Input: dimensioned drawing with shaded views. Units: mm. Origin: part minimum x, y, z. A direction names the side the tool comes from. Coordinates: 2 decimals unless noted, no trailing zeros. Order: outer loops, then holes, each group sorted by start corner. A loop starts at its lowest first (then second) coordinate and runs counter-clockwise, first axis right, second up. Notation, with made-up numbers: (2, 41.25) -> (51, 41.25) arc R31 cw to (51, 75.25) -> close; hole circle Ø3 at (-11.75, -4.75). An arc over 180 degrees is marked (long way). Write item = value, one per line. Start each with the question number.
Item 1: Set-up query: the marked faces 1 and 2. Return all of +Z, -Z, +X, -X, +Y, -Y with unobstructed straight access to the full face (end or side cutting, diameter ignored); none if empty.
Item 2: Section query B-B (x = 36). Output: boundary loops of the cut face in (y, z), then the cut area to 3 significant figures.
Item 3: Ray query, line 1 along Z through (x, y) = (36, 2); line 2 along Y through (x, z) = (2.35, 10). Return the intervals inside material, ascending. Write a range as [from, to].
Item 4: Section query D-D (z = 45). Output: boundary loops of the cut face in (x, y), then the cut area to 3 significant figures.
Item 5: Contact query for flat-ended pins moving along their axis: pin 1 (4 mm diameter, centred on x = 36, z = 40, fed in from +Y) (3 decimals); pin 2 (8.5 mm diameter, centred on y = 36, z = 10, fed in from +X); pin 3 (1 mm diameter, centred on x = 26, z = 39.5, fed in from +Y). Output: stop coordinate, or through.
Item 6: Section query A-A (z = 10). Output: boundary loops of the cut face in (x, y), then the cut area to 3 significant figures.
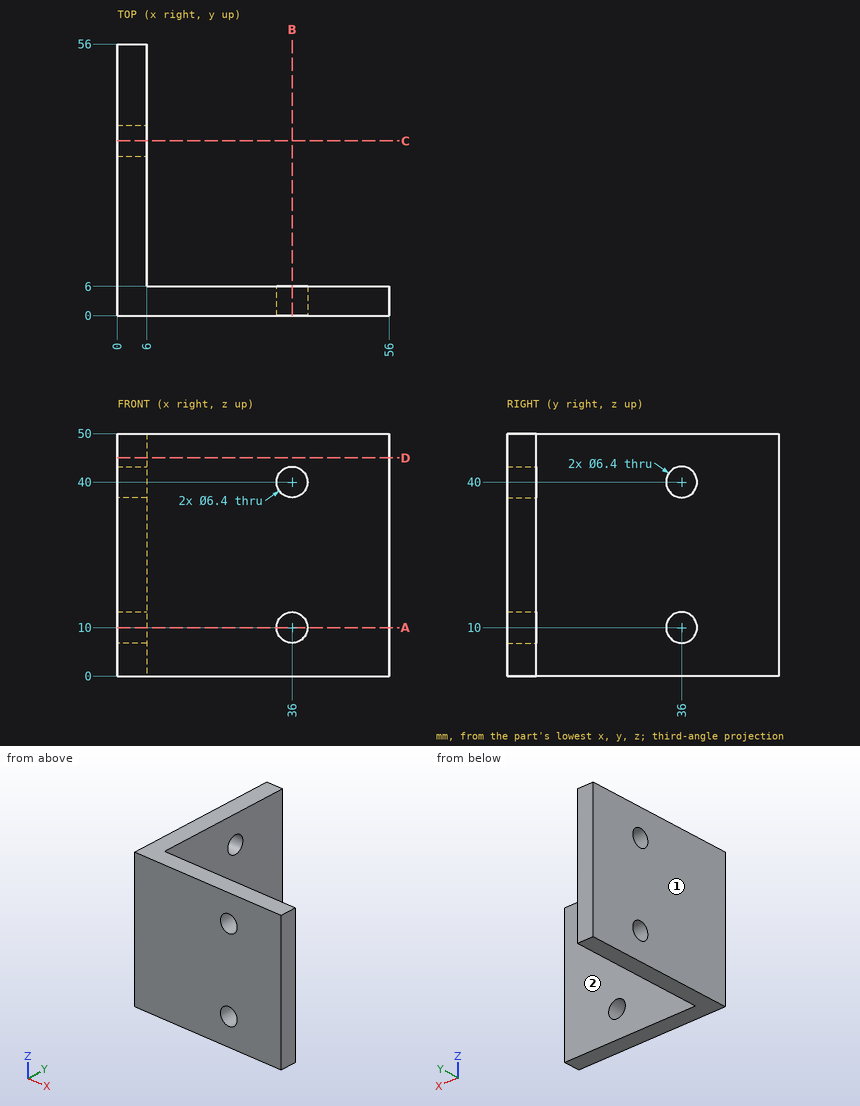
Computed:
q1.face_1 = +Z, -Z, -X, +Y, -Y
q1.face_2 = +Z, -Z, +X, +Y
q2.outline = (0, 0) -> (6, 0) -> (6, 6.8) -> (0, 6.8) -> close; (0, 13.2) -> (6, 13.2) -> (6, 36.8) -> (0, 36.8) -> close; (0, 43.2) -> (6, 43.2) -> (6, 50) -> (0, 50) -> close
q2.area = 223 mm^2
q3.line_1 = [0, 6.8], [13.2, 36.8], [43.2, 50]
q3.line_2 = [0, 32.8], [39.2, 56]
q4.outline = (0, 0) -> (56, 0) -> (56, 6) -> (6, 6) -> (6, 56) -> (0, 56) -> close
q4.area = 636 mm^2
q5.pin_1 = through
q5.pin_2 = 6
q5.pin_3 = 6
q6.outline = (0, 0) -> (32.8, 0) -> (32.8, 6) -> (6, 6) -> (6, 32.8) -> (0, 32.8) -> close; (0, 39.2) -> (6, 39.2) -> (6, 56) -> (0, 56) -> close; (39.2, 0) -> (56, 0) -> (56, 6) -> (39.2, 6) -> close
q6.area = 559 mm^2
